```python
from build123d import *

# Parameters (mm, degrees)
F1_DEPTH = 7
F2_R     = 3.5
F3_DEPTH = 3.5
F4_R     = 3.5
F5_DEPTH = 3.5


with BuildPart() as f1:
    # F0 (on Front) → F1 (new body)
    with BuildSketch(Plane.XZ):
        with BuildLine():
            ThreePointArc((6.839722, -18.510638), (5.92385, -10), (6.839722, -1.489362))
            ThreePointArc((6.839722, -1.489362), (0, 7), (-6.839722, -1.489362))
            ThreePointArc((-6.839722, -1.489362), (-5.92385, -10), (-6.839722, -18.510638))
            ThreePointArc((-6.839722, -18.510638), (0, -27), (6.839722, -18.510638))
        make_face()
    extrude(amount=F1_DEPTH)

    # F2 (on face) → F3 (join)
    with BuildSketch(Plane(origin=(0, 0, 0), x_dir=(-1, 0, 0), z_dir=(0, 1, 0))):
        Circle(F2_R)
        with Locations((0, -20)):
            Circle(F2_R)
    extrude(amount=F3_DEPTH)

    # F4 (on face) → F5 (join)
    with BuildSketch(Plane.XZ.offset(7)):
        Circle(F4_R)
        with Locations((0, -20)):
            Circle(F4_R)
    extrude(amount=F5_DEPTH)


solid = f1.part
```
Design review of the part built by this model. Coordinates are the model's own, in mm. A direction names the side the tool comes from. Give positions to 0.01 mm unless a question says otherwise; leave off trailing zeros. Order: outer loops, then holes, each group sorted by start corner. A loop starts at its lowest first (then second) coordinate and runs counter-clockwise, first axis right, second up. Notation, with made-up numbers: M 23.5,31.25 L 32.5,31.25 A12 ccw 32.5,50.25 Z; hole C 34.5,28 d8. An arc over 180 degrees is marked long. One line per question, with ' | ' between items. Start each with the question number.
Q1. The part is to be moulded in two halves that separate along Z. For faces 4 (the face through (0.46, 1.73, -16.53)), 5 (the face through (0, -7, -10)), 6 (the face through (0, 3.5, 0)), say which applies: +Z half, -Z half, draft (parallel to the pull), parting line (faces both ways), or undercut.
Q2. For L1, parallel to Y at x = 4.5, z = -6; L2, parallel to X at y = -1.5, z = -21.5; L3, parallel to X at y = -6.75, z = -14, list the stretches that pass through material, from the lowest coordinate up. Write a range as [from, to].
Q3. We need section B-B (z = 0). Write out the cut boundary in (x, y).
Q4. Machinability: for faces 1 (the face through (3.233, -8.726, -1.341)), 2 (the face through (-5.924, -3.451, -9.88)), 3 (the face through (0, 0, -10)), which of the approach directions +Z, -Z, +X, -X, +Y, -Y give a long, thin tool a straight path to every point of the face, cutting with its end or side? Answer none if there is none.
Q5. We need section C-C (x = 0). Write out the cut boundary in (y, z), plus the area to 3 significant figures.
Q6. For pin 1 Ø1.5 at (y, z) = (-1.5, -3.5) entering from +X; pin 2 Ø5 at (y, z) = (-4, -12.5) entering from +X; pin 3 Ø4 at (x, y) = (2, -7.5) entering from -Z; pin 4 Ø4 at (x, z) = (3.5, -8.5) entering from +Y, all flat-tipped, find the tip position at first contact; note any pin that passes through.
Q7. We need section D-D (y = -3.75). Write out the cut boundary in (x, z).
Q8. We need section A-A (x = 6.25). Write out the cut boundary in (y, z), plus the area to 3 significant figures.
Returned:
1) face 4: undercut | face 5: undercut | face 6: draft
2) L1: [-7, 0] | L2: [-6.84, 6.84] | L3: [-6.12, 6.12]
3) outline: M -7,-7 L -3.5,-7 L -3.5,-10.5 L 3.5,-10.5 L 3.5,-7 L 7,-7 L 7,0 L 3.5,0 L 3.5,3.5 L -3.5,3.5 L -3.5,0 L -7,0 Z
4) face 1: -Y | face 2: -X, +Y, -Y | face 3: +Y
5) outline: M -10.5,-23.5 L -7,-23.5 L -7,-27 L 0,-27 L 0,-23.5 L 3.5,-23.5 L 3.5,-16.5 L 0,-16.5 L 0,-3.5 L 3.5,-3.5 L 3.5,3.5 L 0,3.5 L 0,7 L -7,7 L -7,3.5 L -10.5,3.5 L -10.5,-3.5 L -7,-3.5 L -7,-16.5 L -10.5,-16.5 Z | area: 336 mm2
6) pin 1: x = 6.59 | pin 2: x = 6.24 | pin 3: z = -27 | pin 4: y = 0
7) outline: M -6.84,-18.51 A7 ccw long 6.84,-18.51 A40 cw 6.84,-1.49 A7 ccw long -6.84,-1.49 A40 cw Z
8) outline: M -7,-23.15 L 0,-23.15 L 0,-15.1 L -7,-15.1 Z; M -7,-4.9 L 0,-4.9 L 0,3.15 L -7,3.15 Z | area: 113 mm2
